The listing builds one solid part. Answer for the finished solid, in the listing's coordinates (mm). A direction names the side the tool comes from. Round coordinates to 2 decimals unless told otherwise and drop trailing zeros. Write each loop counter-clockwise with the first axis right and the second up, starting at its lowest first coordinate (ties: lowest second). Pieces come first, ordered by that corner, then holes.
from build123d import *

# Parameters (mm, degrees)
SKETCH9_R                 = 6.5
BOSS_EXTRUDE3_DEPTH       = 3
BOSS_EXTRUDE4_DEPTH       = 3
FILLET9_R                 = 0.3
FILLET10_R                = 0.3
FILLET11_R                = 0.3
FILLET12_R                = 0.3
CIRPATTERN6_COUNT         = 11
FILLET9_OF_CIRPATTERN6_R  = 0.3
FILLET10_OF_CIRPATTERN6_R = 0.3
FILLET11_OF_CIRPATTERN6_R = 0.3
FILLET12_OF_CIRPATTERN6_R = 0.3
SKETCH11_R                = 1.5
CUT_EXTRUDE1_DEPTH        = 3
SKETCH12_R                = 3
CUT_EXTRUDE2_DEPTH        = 3


with BuildPart() as part:
    # Sketch9 → Boss-Extrude3 (new body)
    with BuildSketch(Plane(origin=(0, 0, 0), x_dir=(0, 0, -1), z_dir=(1, 0, 0))):
        Circle(SKETCH9_R)
    extrude(amount=BOSS_EXTRUDE3_DEPTH)

    # Sketch10 → Boss-Extrude4 (add)
    with BuildSketch(Plane(origin=(3, 0, 0), x_dir=(0, 0, -1), z_dir=(1, 0, 0))):
        Polygon((0, 9.5), (0.75, 9.5), (1.5, 5), (0, 5), (-1.5, 5), (-0.75, 9.5), align=None)
    boss_extrude4 = extrude(amount=-BOSS_EXTRUDE4_DEPTH)

    # Fillet9
    fillet9_edges = [part.edges().sort_by_distance(p)[0] for p in [
        (1.5, 9.5, -0.75),
    ]]
    fillet(fillet9_edges, radius=FILLET9_R)

    # Fillet10
    fillet10_edges = [part.edges().sort_by_distance(p)[0] for p in [
        (1.5, 9.5, 0.75),
    ]]
    fillet(fillet10_edges, radius=FILLET10_R)

    # Fillet11
    fillet11_edges = [part.edges().sort_by_distance(p)[0] for p in [
        (1.5, 6.374542236, -1.270909627),
    ]]
    fillet(fillet11_edges, radius=FILLET11_R)

    # Fillet12
    fillet12_edges = [part.edges().sort_by_distance(p)[0] for p in [
        (1.5, 6.374542236, 1.270909627),
    ]]
    fillet(fillet12_edges, radius=FILLET12_R)

    # CirPattern6: Boss-Extrude4 ×11 about axis
    cirpattern6_axis = Axis((0, 0, 0), (1, 0, 0))
    for i in range(1, CIRPATTERN6_COUNT):
        add(boss_extrude4.rotate(cirpattern6_axis, i * 360 / CIRPATTERN6_COUNT))

    # Fillet9 of CirPattern6
    fillet9_of_cirpattern6_edges = [part.edges().sort_by_distance(p)[0] for p in [
        (1.5, 8.397389175, 4.505147616),
        (1.5, 4.62866662, 8.329942696),
        (1.5, -0.609624882, 9.510039827),
        (1.5, -5.654364792, 7.670766507),
        (1.5, -8.903883832, 3.39607902),
        (1.5, -9.326482667, -1.95683956),
        (1.5, -6.787989153, -6.688475406),
        (1.5, -2.094357045, -9.296567569),
        (1.5, 3.264218627, -8.953065216),
        (1.5, 7.586427949, -5.767027915),
    ]]
    fillet(fillet9_of_cirpattern6_edges, radius=FILLET9_OF_CIRPATTERN6_R)

    # Fillet10 of CirPattern6
    fillet10_of_cirpattern6_edges = [part.edges().sort_by_distance(p)[0] for p in [
        (1.5, 7.586427949, 5.767027915),
        (1.5, 3.264218627, 8.953065216),
        (1.5, -2.094357045, 9.296567569),
        (1.5, -6.787989153, 6.688475406),
        (1.5, -9.326482667, 1.95683956),
        (1.5, -8.903883832, -3.39607902),
        (1.5, -5.654364792, -7.670766507),
        (1.5, -0.609624882, -9.510039827),
        (1.5, 4.62866662, -8.329942696),
        (1.5, 8.397389175, -4.505147616),
    ]]
    fillet(fillet10_of_cirpattern6_edges, radius=FILLET10_OF_CIRPATTERN6_R)

    # Fillet11 of CirPattern6
    fillet11_of_cirpattern6_edges = [part.edges().sort_by_distance(p)[0] for p in [
        (1.5, 6.049711796, 2.377180512),
        (1.5, 3.804140606, 5.270532634),
        (1.5, 0.350781652, 6.490527885),
        (1.5, -3.213947997, 5.649826393),
        (1.5, -5.758271867, 3.01534494),
        (1.5, -6.474385104, -0.576487225),
        (1.5, -5.134926817, -3.98528877),
        (1.5, -2.165165547, -6.128789289),
        (1.5, 1.492020486, -6.326442513),
        (1.5, 4.675500556, -4.515494939),
    ]]
    fillet(fillet11_of_cirpattern6_edges, radius=FILLET11_OF_CIRPATTERN6_R)

    # Fillet12 of CirPattern6
    fillet12_of_cirpattern6_edges = [part.edges().sort_by_distance(p)[0] for p in [
        (1.5, 4.675500556, 4.515494939),
        (1.5, 1.492020486, 6.326442513),
        (1.5, -2.165165547, 6.128789289),
        (1.5, -5.134926817, 3.98528877),
        (1.5, -6.474385104, 0.576487225),
        (1.5, -5.758271867, -3.01534494),
        (1.5, -3.213947997, -5.649826393),
        (1.5, 0.350781652, -6.490527885),
        (1.5, 3.804140606, -5.270532634),
        (1.5, 6.049711796, -2.377180512),
    ]]
    fillet(fillet12_of_cirpattern6_edges, radius=FILLET12_OF_CIRPATTERN6_R)

    # Sketch11 → Cut-Extrude1 (cut)
    with BuildSketch(Plane(origin=(3, 0, 0), x_dir=(0, 0, -1), z_dir=(1, 0, 0))):
        with Locations((0, 4.75)):
            Circle(SKETCH11_R)
        with Locations((4.75, 0)):
            Circle(SKETCH11_R)
        with Locations((-4.75, 0)):
            Circle(SKETCH11_R)
        with Locations((0, -4.75)):
            Circle(SKETCH11_R)
    extrude(amount=-CUT_EXTRUDE1_DEPTH, mode=Mode.SUBTRACT)

    # Sketch12 → Cut-Extrude2 (cut)
    with BuildSketch(Plane(origin=(3, 0, 0), x_dir=(0, 0, -1), z_dir=(1, 0, 0))):
        Circle(SKETCH12_R)
    extrude(amount=-CUT_EXTRUDE2_DEPTH, mode=Mode.SUBTRACT)


solid = part.part
1. Section C-C on x = 0.85 is taken. Give the number of separate pieces and of enclosed holes in the cut face, plus the area to 3 significant figures.
Geometry says:
separate pieces: 1
enclosed holes: 5
area: 143 mm2
2. A tool of negligible diameter and unlimited length cuts with its end or side. For faces 1 (the face through (1.5, -7.3, 3.2)), 2 (the face through (1.52, 7.19, -3.41)), 3 (the face through (1.521, 6.09, 5.124)), from which of +Z, -Z, +X, -X, +Y, -Y can it reach the whole face along a straight path? Write none if from no direction.
Geometry says:
face 1: +X, -X
face 2: +X, -X, +Y
face 3: +Z, +X, -X
3. Given pin 1 (1.5 mm diameter, centred on y = 0.5, z = -1, fed in from +X), flat-ended and moving along its own axis, determine where the tip first touches the part or whether it passes through.
Geometry says:
pin 1: passes through
4. Section A-A on y = 0 is taken. Determine the outline of the cut face in (x, z).
Geometry says:
outline: (0, -7.59) - (3, -7.59) - (3, -6.25) - (0, -6.25) - close; (0, -3.25) - (3, -3.25) - (3, -3) - (0, -3) - close; (0, 3) - (3, 3) - (3, 3.25) - (0, 3.25) - close; (0, 6.25) - (3, 6.25) - (3, 7.59) - (0, 7.59) - close
5. Section B-B on y = -4.75 is taken. Determine the outline of the cut face in (x, z), plus the area to 3 significant figures.
Geometry says:
outline: (0, -6.92) - (3, -6.92) - (3, -1.5) - (0, -1.5) - close; (0, 1.5) - (3, 1.5) - (3, 6.92) - (0, 6.92) - close
area: 32.5 mm2
6. Straight lines are drawn through the part: line 1 along Y through (x, z) = (0.95, 0); line 2 along Z through (x, y) = (0.9, 7.75); line 3 along Y through (x, z) = (1.45, 4.75). For each, find the intervals that lie inside material, in ascending order.
Geometry says:
line 1: y = -6.5 to -6.25, -3.25 to -3, 3 to 3.25, 6.25 to 9.5
line 2: z = -5.51 to -3.92, -1.04 to 1.04, 3.92 to 5.51
line 3: y = -5.6 to -1.5, 1.5 to 4.44, 5.22 to 8.24
7. For a pull along Y with two mould halves and no side action, classify faces 4 (the face through (1.52, 2.35, 7.6)), 5 (the face through (1.5, 4.8, 1.5)), 6 (the face through (1.521, -1.359, -9.402)), 7 (the face through (1.52, 3.95, 8.64)) as released by +Y, released by -Y, zero draft, split by the parting line, or undercut.
Geometry says:
face 4: undercut
face 5: undercut
face 6: released by -Y
face 7: released by +Y
